```python
from build123d import *

# Parameters (mm, degrees)
CYLINDER_R     = 1.7
CYLINDER_DEPTH = 10


with BuildPart() as cono:
    # Cone → Cone (revolve)
    with BuildSketch(Plane.XZ):
        Polygon((0, 0), (3, 0), (5, 3), (0, 3), align=None)
    revolve(axis=Axis((0, 0, 0), (0, 0, 1)))


with BuildPart() as fusion:
    # Cone001 → Cone001 (revolve)
    with BuildSketch(Plane(origin=(0, 0, 0), x_dir=(1, 0, 0), z_dir=(0, 1, 0))):
        Polygon((0, 0), (3, 0), (5, 3), (0, 3), align=None)
    revolve(axis=Axis((0, 0, 0), (0, 0, -1)))

    # Fusion: union Cono
    add(cono.part)


with BuildPart() as fusion001002:
    # Cylinder → Cylinder (new body)
    with BuildSketch(Plane.XY.offset(-5)):
        Circle(CYLINDER_R)
    extrude(amount=CYLINDER_DEPTH)

    # Fusion001002: union Fusion
    add(fusion.part)


solid = fusion001002.part
```
The listing builds one solid part. Answer for the finished solid, in the listing's coordinates (mm). A direction names the side the tool comes from. Coordinates: 2 decimals unless noted, no trailing zeros. Loops run counter-clockwise (first coordinate to the right, second up) from the corner with the lowest first, then second, coordinate; pieces in that order, holes last. Notation, with made-up numbers: (28.25, -1) - (75.25, -1) arc R29 ccw to (75.25, 19) - close; hole circle Ø7 at (33.25, -18.5). An arc over 180 degrees is marked (long way). Use a Markdown table: item, result. Add a question column.
1) The mould has two halves that part along Z. Classify faces 4 (the cylindrical face through (-0.37, -1.66, -4.01)), 5 (the flat face through (2, 0, -3)), 6 (the conical face through (-0.68, 3.05, -0.19)): released by +Z, released by -Z, zero draft, split by the parting line, or undercut.
2) Given pin 1 (1.5 mm diameter, centred on x = -0.5, z = 1, fed in from -Y); pin 2 (1.5 mm diameter, centred on x = -1, z = 3.5, fed in from -Y); pin 3 (1 mm diameter, centred on x = -2, y = 4, fed in from -Z), each flat-ended and moving along its own axis, determine where each tip first touches the part or whether it passes through.
3) Find the intervals of material crossed by line 1 (Z direction, x = 3.75, y = 3); line 2 (Z direction, x = 0.5, y = 3.5); line 3 (Z direction, x = -2, y = -1), in increasing order.
4) For faces 1 (the conical face through (-0.68, -3.05, 0.19)), 2 (the flat face through (0, 0, -5)), 3 (the flat face through (2, 0, 3)), determine the directions among +Z, -Z, +X, -X, +Y, -Y from which every point of the face is accessible in a straight line to the end or side of a thin tool.
5) The part is cut by section A-A, the plane y = 0. Give the vertices of the cut face in (x, z), and give its area (3 significant figures).
6) The part is cut by section C-C, the plane z = -0.25. Give the vertices of the cut face in (x, y), and give its area (3 significant figures).
7) The part is cut by section D-D, the plane z = 2.5. Give the vertices of the cut face in (x, y), and give its area (3 significant figures).
Here are the results:
| question | item | result |
|---|---|---|
| 1 | face 4 | zero draft |
| 1 | face 5 | released by -Z |
| 1 | face 6 | undercut |
| 2 | pin 1 | stops at y = -4.14 |
| 2 | pin 2 | stops at y = -4.98 |
| 2 | pin 3 | stops at z = -3 |
| 3 | line 1 | z = -3 to -2.7, 2.7 to 3 |
| 3 | line 2 | z = -3 to -0.8, 0.8 to 3 |
| 3 | line 3 | z = -3 to 3 |
| 4 | face 1 | none |
| 4 | face 2 | -Z, +X, -X, +Y, -Y |
| 4 | face 3 | +Z |
| 5 | outline | (-5, -3) - (-1.7, -3) - (-1.7, -5) - (1.7, -5) - (1.7, -3) - (5, -3) - (3, 0) - (5, 3) - (1.7, 3) - (1.7, 5) - (-1.7, 5) - (-1.7, 3) - (-5, 3) - (-3, 0) - close |
| 5 | area | 61.6 mm^2 |
| 6 | outline | circle Ø6.33 at (0, 0) |
| 6 | area | 31.5 mm^2 |
| 7 | outline | circle Ø9.33 at (0, 0) |
| 7 | area | 68.4 mm^2 |
